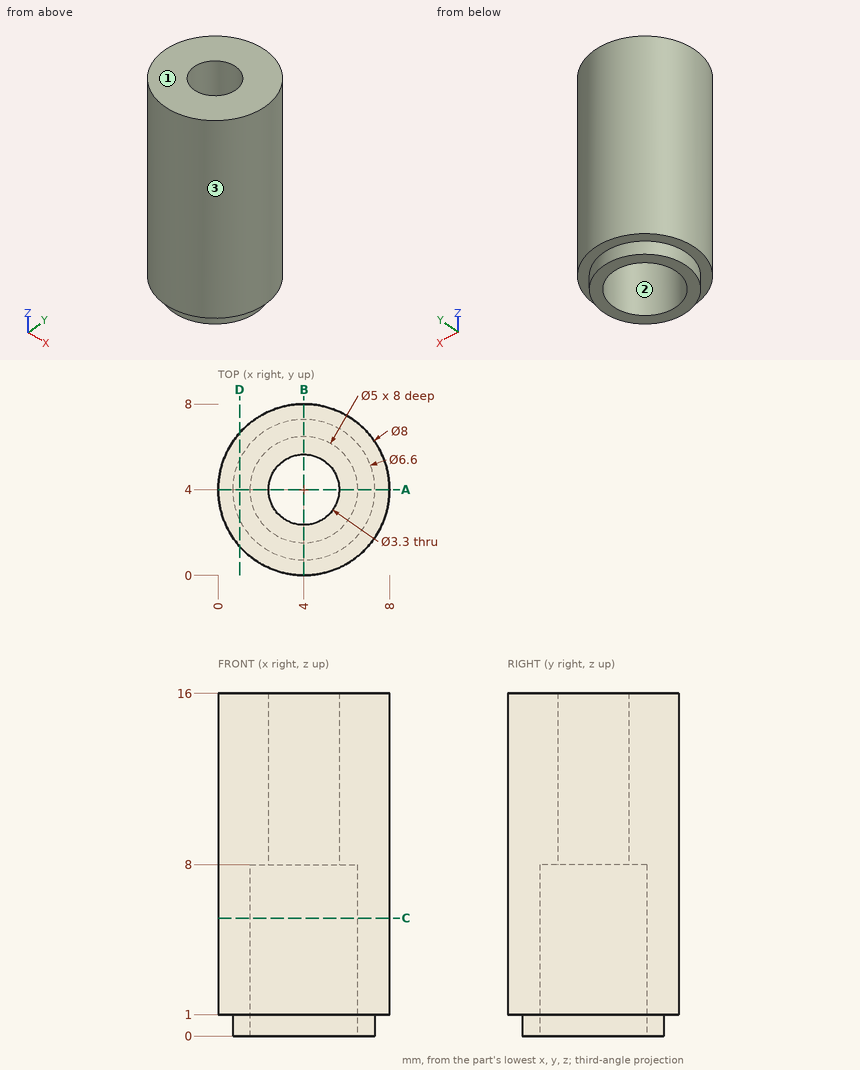
For this review, use the dimensioned drawing (mm, ordinates from the lowest corner) and the shaded views. Round coordinates to 2 decimals unless told otherwise and drop trailing zeros. Write each loop counter-clockwise with the first axis right and the second up, starting at its lowest first coordinate (ties: lowest second). Pieces come first, ordered by that corner, then holes. Notation, with made-up numbers: (55, 46) - (69, 46) arc R23 cw to (69, 71) - close; hole circle Ø9 at (-26.75, -37.5). An arc over 180 degrees is marked (long way). Use a Markdown table: item, result.
Q1. The part is to be moulded in two halves that separate along Y. For the marked faces 1, 2 and 3, say which applies: pulls with the +Y half, pulls with the -Y half, needs draft (parallel to the pull), parting line crosses it, or undercut.
Derived:
| item | result |
|---|---|
| face 1 | needs draft |
| face 2 | undercut |
| face 3 | parting line crosses it |
Q2. We need section D-D (x = 1). Give the boundary of the cut face in (y, z).
Derived:
| item | result |
|---|---|
| outline | (1.35, 1) - (2.63, 1) - (2.63, 0) - (5.37, 0) - (5.37, 1) - (6.65, 1) - (6.65, 16) - (1.35, 16) - close |
Q3. We need section A-A (y = 4). Give the boundary of the cut face in (x, z).
Derived:
| item | result |
|---|---|
| outline | (0, 1) - (0.7, 1) - (0.7, 0) - (1.5, 0) - (1.5, 8) - (2.35, 8) - (2.35, 16) - (0, 16) - close; (5.65, 8) - (6.5, 8) - (6.5, 0) - (7.3, 0) - (7.3, 1) - (8, 1) - (8, 16) - (5.65, 16) - close |
Q4. Wall thickness on line 1 along Y through (x, z) = (4, 6); line 2 along Y through (x, z) = (4, 12.75); line 3 along Z through (x, y) = (2, 4.5): over which ranges is each line inside the solid? List them lowest first.
Derived:
| item | result |
|---|---|
| line 1 | y = 0 to 1.5, 6.5 to 8 |
| line 2 | y = 0 to 2.35, 5.65 to 8 |
| line 3 | z = 8 to 16 |
Q5. We need section C-C (z = 5.5). Give the boundary of the cut face in (x, y).
Derived:
| item | result |
|---|---|
| outline | circle Ø8 at (4, 4); hole circle Ø5 at (4, 4) |
Q6. Clearance check with flat-ended pins moving along their axes: pin 1 (1.5 mm diameter, centred on x = 3.5, y = 4.5, fed in from -Z); pin 2 (1.5 mm diameter, centred on x = 6.5, z = 13.5, fed in from +Y); pin 3 (1.5 mm diameter, centred on x = 5.5, y = 5.5, fed in from -Z); pin 4 (2 mm diameter, centred on y = 1.5, z = 2.5, fed in from +X). State where each tip first meets the part, or that it passes through.
Derived:
| item | result |
|---|---|
| pin 1 | passes through |
| pin 2 | stops at y = 7.6 |
| pin 3 | stops at z = 0 |
| pin 4 | stops at x = 7.71 |
